The listing builds one solid part. Answer for the finished solid, in the listing's coordinates (mm). Give positions to 0.01 mm unless a question says otherwise; leave off trailing zeros. Write each loop counter-clockwise with the first axis right and the second up, starting at its lowest first coordinate (ties: lowest second). Pieces come first, ordered by that corner, then holes. Notation, with made-up numbers: M -16,86 L 28,86 A32 cw 28,122 Z; hole C 83,10 d7. An arc over 180 degrees is marked long. Answer as a JSON object with one key per item and string values.
```python
from build123d import *

# Parameters (mm, degrees)
SKETCH1_W          = 7.5
SKETCH1_H          = 204
SKETCH2_W          = 3
SKETCH2_H          = 3
CUT_EXTRUDE1_DEPTH = 18
SKETCH3_W          = 3
SKETCH3_H          = 3
CUT_EXTRUDE2_DEPTH = 15


with BuildPart() as part:
    # Sketch1 → Revolve1 (revolve)
    with BuildSketch(Plane.XY, mode=Mode.PRIVATE) as revolve1_sk:
        with Locations((3.75, 102)):
            Rectangle(SKETCH1_W, SKETCH1_H)
    revolve(revolve1_sk.sketch.rotate(Axis((0, 204, 0), (0, -1, 0)), 180), axis=Axis((0, 204, 0), (0, -1, 0)))

    # Sketch2 → Cut-Extrude1 (cut)
    with BuildSketch(Plane(origin=(0, 187, 0), x_dir=(1, 0, 0), z_dir=(0, 1, 0))):
        with Locations((0, 7.5)):
            Rectangle(SKETCH2_W, SKETCH2_H)
    extrude(amount=-CUT_EXTRUDE1_DEPTH, mode=Mode.SUBTRACT)

    # Sketch3 → Cut-Extrude2 (cut)
    with BuildSketch(Plane(origin=(0, 104, 0), x_dir=(-1, 0, 0), z_dir=(0, -1, 0))):
        with Locations((0, 7.5)):
            Rectangle(SKETCH3_W, SKETCH3_H)
    extrude(amount=CUT_EXTRUDE2_DEPTH, mode=Mode.SUBTRACT)


solid = part.part
```
1. The mould has two halves that part along Z. Classify faces 1 (the cylindrical face through (1.63, 103.43, 7.32)), 2 (the flat face through (0, 0, 0)): released by +Z, released by -Z, zero draft, split by the parting line, or undercut.
Verdict:
{"face 1": "split by the parting line", "face 2": "zero draft"}
2. A cutting plane is placed at A-A, the plane y = 69.5. Give the vertices of the cut face in (x, z).
Verdict:
{"outline": "C 0,0 d15"}
3. Consider line 1 along X through (y, z) = (149.5, 0.5); line 2 along Z through (x, y) = (0.5, 169.5); line 3 along X through (y, z) = (66.5, -3.25). Determine where each line is inside the solid, lowest interval first.
Verdict:
{"line 1": "x = -7.48 to 7.48", "line 2": "z = -6 to 7.48", "line 3": "x = -6.76 to 6.76"}
4. Flat-ended cylindrical pins translate along their axes: pin 1 (5 mm diameter, centred on y = 108.5, z = 5.5, fed in from -X); pin 2 (1.5 mm diameter, centred on y = 174, z = -7, fed in from -X); pin 3 (2 mm diameter, centred on x = 4.5, z = 1.5, fed in from -Y); pin 4 (2.5 mm diameter, centred on x = 0, y = 93.5, fed in from -Z). Find the tip coordinate at first contact, or state that the pin passes through.
Verdict:
{"pin 1": "stops at x = -6.87", "pin 2": "stops at x = -4.15", "pin 3": "stops at y = 0", "pin 4": "stops at z = -6"}
5. A cutting plane is placed at C-C, the plane y = 102. Give the vertices of the cut face in (x, z).
Verdict:
{"outline": "M -1.5,-7.35 L -1.5,-6 L 1.5,-6 L 1.5,-7.35 A7.5 ccw long Z"}
6. A cutting plane is placed at B-B, the plane z = 3.5. Give the vertices of the cut face in (x, y).
Verdict:
{"outline": "M -6.63,0 L 6.63,0 L 6.63,204 L -6.63,204 Z"}
